Input: dimensioned drawing with shaded views. Units: mm. Origin: part minimum x, y, z. A direction names the side the tool comes from. Give positions to 0.01 mm unless a question says otherwise; leave off trailing zeros. Loops run counter-clockwise (first coordinate to the right, second up) from the corner with the lowest first, then second, coordinate; pieces in that order, holes last. Notation, with made-up numbers: (-19.5, 80) -> (23.5, 80) arc R16 ccw to (23.5, 90) -> close; hole circle Ø7 at (26, -17.75). An arc over 180 degrees is marked (long way). Answer in a Markdown table with one row per item. Add a question column.
1) Section query A-A (x = 8.5). Return the cut outline in (y, z).
2) Section query B-B (z = 10.25). Return the cut outline in (x, y).
3) Draft query along X for the marked faces 4, 5 and 6. Return one class per face: +X half, -X half, draft (parallel to the pull), parting line (faces both ways), or undercut.
4) Section query C-C (y = 0.5). Return the cut outline in (x, z).
5) Line query: line 1 (X direction, y = 0.7, z = 10.25); line 2 (Z direction, x = 9.5, y = 2.7). Output: solid intervals per line, ascending. Write a range as from..to.
6) Section query D-D (x = 4.75). Return the cut outline in (y, z).
7) First-contact query: P1, Ø0.9, axis at y = 1.5, z = 10, coming from the +X side; P2, Ø0.9, axis at y = 1.5, z = 10.5, coming from the -X side; P3, Ø0.6, axis at x = 6, y = 3, coming from the -Z side. Flat tips, straight axial feed; report the tip coordinate or a pass-through.
8) Access query for the marked faces 1, 2 and 3. Directions: +Z, -Z, +X, -X, +Y, -Y. A direction counts if a zero-diameter tool reaches every point of the face in a straight line with its end or side. Return the directions, or none.
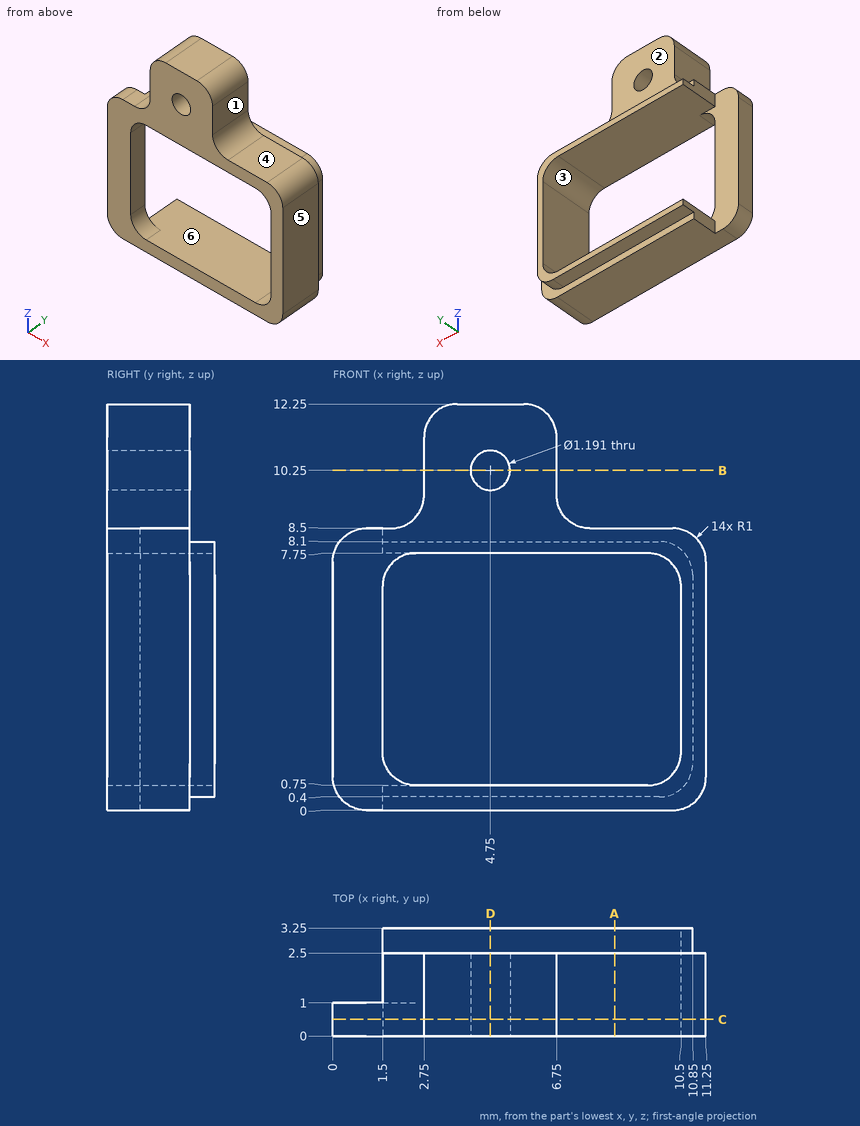
Evaluation:
| question | item | result |
|---|---|---|
| 1 | outline | (0, 0) -> (2.5, 0) -> (2.5, 0.4) -> (3.25, 0.4) -> (3.25, 0.75) -> (0, 0.75) -> close; (0, 7.75) -> (3.25, 7.75) -> (3.25, 8.1) -> (2.5, 8.1) -> (2.5, 8.5) -> (0, 8.5) -> close |
| 2 | outline | (2.75, 0) -> (4.15, 0) -> (4.15, 2.5) -> (2.75, 2.5) -> close; (5.35, 0) -> (6.75, 0) -> (6.75, 2.5) -> (5.35, 2.5) -> close |
| 3 | face 4 | draft |
| 3 | face 5 | +X half |
| 3 | face 6 | undercut |
| 4 | outline | (0, 1) arc R1 ccw to (1, 0) -> (10.25, 0) arc R1 ccw to (11.25, 1) -> (11.25, 7.5) arc R1 ccw to (10.25, 8.5) -> (7.75, 8.5) arc R1 cw to (6.75, 9.5) -> (6.75, 11.25) arc R1 ccw to (5.75, 12.25) -> (3.75, 12.25) arc R1 ccw to (2.75, 11.25) -> (2.75, 9.5) arc R1 cw to (1.75, 8.5) -> (1, 8.5) arc R1 ccw to (0, 7.5) -> close; hole (1.5, 1.75) arc R1 ccw to (2.5, 0.75) -> (9.5, 0.75) arc R1 ccw to (10.5, 1.75) -> (10.5, 6.75) arc R1 ccw to (9.5, 7.75) -> (2.5, 7.75) arc R1 ccw to (1.5, 6.75) -> close; hole circle Ø1.19 at (4.75, 10.25) |
| 5 | line 1 | 2.75..4.15, 5.35..6.75 |
| 5 | line 2 | 0.4..0.75, 7.75..8.1 |
| 6 | outline | (0, 0) -> (2.5, 0) -> (2.5, 0.4) -> (3.25, 0.4) -> (3.25, 0.75) -> (0, 0.75) -> close; (0, 7.75) -> (3.25, 7.75) -> (3.25, 8.1) -> (2.5, 8.1) -> (2.5, 9.65) -> (0, 9.65) -> close; (0, 10.85) -> (2.5, 10.85) -> (2.5, 12.25) -> (0, 12.25) -> close |
| 7 | P1 | x = 6.75 |
| 7 | P2 | x = 2.75 |
| 7 | P3 | z = 0.4 |
| 8 | face 1 | +Z, +X, +Y, -Y |
| 8 | face 2 | +X, +Y |
| 8 | face 3 | +Y, -Y |
